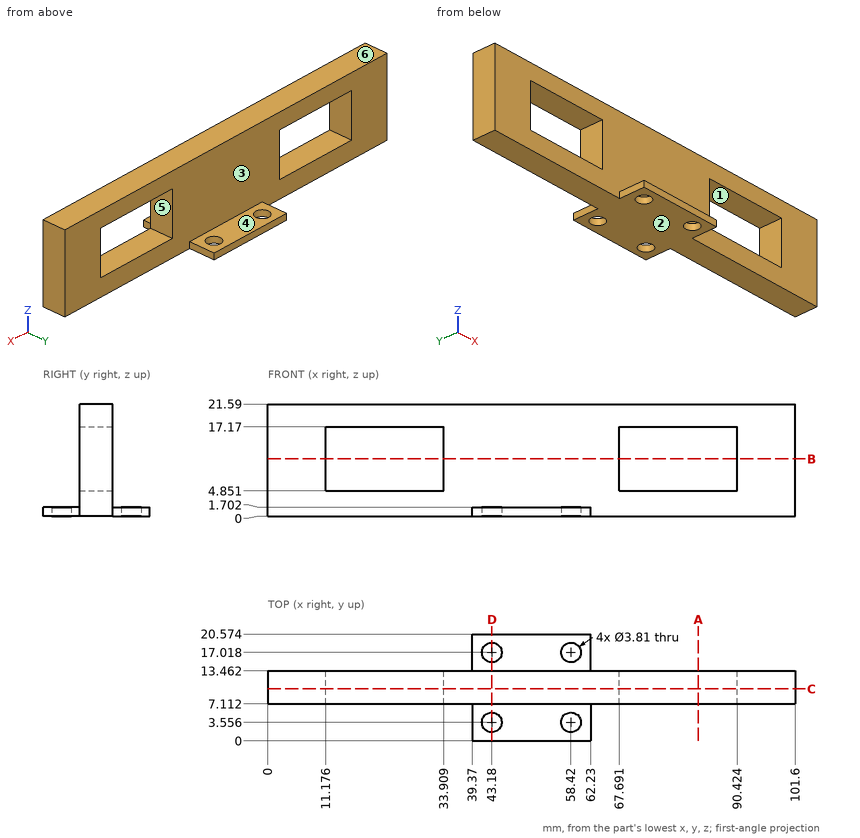
Verification items for this drawing (mm, ordinates from the low corner). A direction names the side the tool comes from. Coordinates: 2 decimals unless noted, no trailing zeros. Write each loop counter-clockwise with the first axis right and the second up, starting at its lowest first coordinate (ties: lowest second). Pieces come first, ordered by that corner, then holes. Notation, with made-up numbers: M -0.75,58 L 46.25,58 A26 ccw 46.25,76 Z; hole C 65,42.25 d10. An arc over 180 degrees is marked long. Answer as a JSON object with one key per item and string values. Group by question number.
(1) Cross-section at D-D, the plane x = 43.18. Record the cut outline in (y, z), and give its area (3 significant figures).
(2) Release check for a two-part mould opening along Z. For the marked faces 1, 2 and 3 record: +Z half, -Z half, draft (parallel to the pull), parting line (faces both ways), or undercut.
(3) Tool access check on the marked faces 4, 5 and 6. Record the directions out of +Z, -Z, +X, -X, +Y, -Y that give a thin tool (end or side, any length) a straight path to the whole face; none if there is none.
(4) Cross-section at A-A, the plane x = 83. Record the cut outline in (y, z).
(5) Material ranges on line 1 (X direction, y = 9, z = 6.5); line 2 (Y direction, x = 58.42, z = 1.3); line 3 (Z direction, x = 28.5, y = 11), recorded low to high.
(6) Gauge pin test, flat ends, axial feed: pin 1 (12 mm diameter, centred on x = 90.5, z = 13.5, fed in from +Y); pin 2 (6 mm diameter, centred on x = 58.42, y = 17.018, fed in from +Z); pin 3 (1.9 mm diameter, centred on y = 15.5, z = 1, fed in from -X). Record the tip position at first contact, or that the pin passes through.
(7) Cross-section at C-C, the plane y = 10. Record the cut outline in (x, z), and give its area (3 significant figures).
(8) Cross-section at B-B, the plane z = 11. Record the cut outline in (x, y).
Reply:
{
 "1": {"outline": "M 0,0 L 1.65,0 L 1.65,1.7 L 0,1.7 Z; M 5.46,0 L 15.11,0 L 15.11,1.7 L 13.46,1.7 L 13.46,21.59 L 7.11,21.59 L 7.11,1.7 L 5.46,1.7 Z; M 18.92,0 L 20.57,0 L 20.57,1.7 L 18.92,1.7 Z", "area": "148 mm²"},
 "2": {"face 1": "undercut", "face 2": "-Z half", "face 3": "draft"},
 "3": {"face 4": "+Z, +X, -X, +Y", "face 5": "+Y, -Y", "face 6": "+Z, +X, -X, +Y, -Y"},
 "4": {"outline": "M 7.11,0 L 13.46,0 L 13.46,4.85 L 7.11,4.85 Z; M 7.11,17.17 L 13.46,17.17 L 13.46,21.59 L 7.11,21.59 Z"},
 "5": {"line 1": "0 to 11.18, 33.91 to 67.69, 90.42 to 101.6", "line 2": "0 to 1.65, 5.46 to 15.11, 18.92 to 20.57", "line 3": "0 to 4.85, 17.17 to 21.59"},
 "6": {"pin 1": "y = 13.46", "pin 2": "z = 1.7", "pin 3": "x = 39.37"},
 "7": {"outline": "M 0,0 L 101.6,0 L 101.6,21.59 L 0,21.59 Z; hole M 11.18,4.85 L 33.91,4.85 L 33.91,17.17 L 11.18,17.17 Z; hole M 67.69,4.85 L 90.42,4.85 L 90.42,17.17 L 67.69,17.17 Z", "area": "1,630 mm²"},
 "8": {"outline": "M 0,7.11 L 11.18,7.11 L 11.18,13.46 L 0,13.46 Z; M 33.91,7.11 L 67.69,7.11 L 67.69,13.46 L 33.91,13.46 Z; M 90.42,7.11 L 101.6,7.11 L 101.6,13.46 L 90.42,13.46 Z"}
}
